Input: part model. Units: mm. Frame: model coordinates. Face numbers are marked on the shaded views. A direction names the side the tool comes from. Coordinates: 2 decimals unless noted, no trailing zeros. Loops run counter-clockwise (first coordinate to the right, second up) from the corner with the lowest first, then second, coordinate; pieces in that order, holes last. Notation, with made-up numbers: (37, 79.25) -> (58, 79.25) arc R11 ccw to (58, 83.25) -> close; hole circle Ø11 at (88.25, 81.5). An arc over 180 degrees is marked (long way). Answer as a JSON object with one key per item and string values.
from build123d import *

# Parameters (mm, degrees)
CROQUIS1_W                = 30
CROQUIS1_H                = 30
SALIENTE_EXTRUIR1_DEPTH   = 3
CROQUIS2_W                = 15
CROQUIS2_H                = 30
SALIENTE_EXTRUIR3_DEPTH   = 3
SALIENTE_EXTRUIR3_2_DEPTH = 3
CROQUIS3_W                = 30
CROQUIS3_H                = 30
SALIENTE_EXTRUIR4_DEPTH   = 3
SALIENTE_EXTRUIR5_DEPTH   = 3
CORTAR_EXTRUIR1_DEPTH     = 6
SALIENTE_EXTRUIR8_DEPTH   = 11
CROQUIS7_W                = 30
CROQUIS7_H                = 3.175
CORTAR_EXTRUIR3_DEPTH     = 18.542
CROQUIS9_W                = 60
CROQUIS9_H                = 0.175
SALIENTE_EXTRUIR9_DEPTH   = 11
CROQUIS10_W               = 90
CROQUIS10_H               = 5
CORTAR_EXTRUIR5_DEPTH     = 93
CROQUIS11_W               = 30
CROQUIS11_H               = 3.175
SALIENTE_EXTRUIR10_DEPTH  = 11
CROQUIS12_W               = 60
CROQUIS12_H               = 0.175
CORTAR_EXTRUIR6_DEPTH     = 11
CROQUIS13_W               = 30
CROQUIS13_H               = 5
CORTAR_EXTRUIR7_DEPTH     = 10
SALIENTE_EXTRUIR11_DEPTH  = 5


with BuildPart() as part:
    # Croquis1 → Saliente-Extruir1 (new body)
    with BuildSketch(Plane(origin=(0, 0, 0), x_dir=(1, 0, 0), z_dir=(0, 1, 0))):
        Rectangle(CROQUIS1_W, CROQUIS1_H)
    extrude(amount=SALIENTE_EXTRUIR1_DEPTH)



with BuildPart() as body_2:
    # Croquis2 → Saliente-Extruir3 (new body)
    with BuildSketch(Plane(origin=(0, 3, 0), x_dir=(1, 0, 0), z_dir=(0, 1, 0))):
        with Locations((-22.5, -30)):
            Rectangle(CROQUIS2_W, CROQUIS2_H)
    extrude(amount=-SALIENTE_EXTRUIR3_DEPTH)


with BuildPart() as body_3:
    # Croquis2 → Saliente-Extruir3 2 (new body)
    with BuildSketch(Plane(origin=(0, 3, 0), x_dir=(1, 0, 0), z_dir=(0, 1, 0))):
        with Locations((22.5, -30)):
            Rectangle(CROQUIS2_W, CROQUIS2_H)
    extrude(amount=-SALIENTE_EXTRUIR3_2_DEPTH)


with BuildPart() as part_1:
    add(part.part)

    add(body_2.part)  # Saliente-Extruir4 merges body 2

    add(body_3.part)  # Saliente-Extruir4 merges body 3
    # Croquis3 → Saliente-Extruir4 (add)
    with BuildSketch(Plane(origin=(0, 3, 0), x_dir=(1, 0, 0), z_dir=(0, 1, 0))):
        with Locations((0, -30)):
            Rectangle(CROQUIS3_W, CROQUIS3_H)
    extrude(amount=-SALIENTE_EXTRUIR4_DEPTH)

    # Croquis4 → Saliente-Extruir5 (add)
    with BuildSketch(Plane(origin=(0, 3, 0), x_dir=(1, 0, 0), z_dir=(0, 1, 0))):
        Polygon((-30, 0), (-45, 0), (-45, -60), (45, -60), (45, 0), (30, 0), (30, 30), (-30, 30), align=None)
    extrude(amount=SALIENTE_EXTRUIR5_DEPTH)

    # Croquis5 → Cortar-Extruir1 (cut)
    with BuildSketch(Plane(origin=(0, 0, 0), x_dir=(-1, 0, 0), z_dir=(0, -1, 0))):
        Polygon((30, -45), (30, -15), (15, -15), (15, 15), (-15, 15), (-15, -15), (-30, -15), (-30, -45), align=None)
    extrude(amount=-CORTAR_EXTRUIR1_DEPTH, mode=Mode.SUBTRACT)

    # Croquis6 → Saliente-Extruir8 (add)
    with BuildSketch(Plane(origin=(0, 3, 0), x_dir=(-1, 0, 0), z_dir=(0, -1, 0))):
        with BuildLine():
            Line((37.5, 0), (45, 0))
            Line((45, 0), (45, -60))
            Line((45, -60), (-45, -60))
            Line((-45, -60), (-45, 0))
            Line((-45, 0), (-37.5, 0))
            ThreePointArc((-37.5, 0), (-32.196699141, 2.196699141), (-30, 7.5))
            Line((-30, 7.5), (-30, 30))
            Line((-30, 30), (30, 30))
            Line((30, 30), (30, 7.5))
            ThreePointArc((30, 7.5), (32.196699141, 2.196699141), (37.5, 0))
        make_face()
        Polygon((15, 15), (15, -15), (30, -15), (30, -45), (-30, -45), (-30, -15), (-15, -15), (-15, 15), align=None, mode=Mode.SUBTRACT)
    extrude(amount=-SALIENTE_EXTRUIR8_DEPTH)

    # Croquis7 → Cortar-Extruir3 (cut)
    with BuildSketch(Plane(origin=(0, 14, 0), x_dir=(1, 0, 0), z_dir=(0, 1, 0))):
        with Locations((0, 16.5875)):
            Rectangle(CROQUIS7_W, CROQUIS7_H)
    extrude(amount=-CORTAR_EXTRUIR3_DEPTH, mode=Mode.SUBTRACT)

    # Croquis9 → Saliente-Extruir9 (add)
    with BuildSketch(Plane(origin=(0, 14, 0), x_dir=(1, 0, 0), z_dir=(0, 1, 0))):
        with Locations((0, 30.0875)):
            Rectangle(CROQUIS9_W, CROQUIS9_H)
    extrude(amount=-SALIENTE_EXTRUIR9_DEPTH)

    # Croquis10 → Cortar-Extruir5 (cut)
    with BuildSketch(Plane.XY.offset(60)):
        with Locations((0, 5.5)):
            Rectangle(CROQUIS10_W, CROQUIS10_H)
    extrude(amount=-CORTAR_EXTRUIR5_DEPTH, mode=Mode.SUBTRACT)

    # Croquis11 → Saliente-Extruir10 (add)
    with BuildSketch(Plane(origin=(0, 14, 0), x_dir=(1, 0, 0), z_dir=(0, 1, 0))):
        with Locations((0, 16.5875)):
            Rectangle(CROQUIS11_W, CROQUIS11_H)
    extrude(amount=-SALIENTE_EXTRUIR10_DEPTH)

    # Croquis12 → Cortar-Extruir6 (cut)
    with BuildSketch(Plane(origin=(0, 14, 0), x_dir=(1, 0, 0), z_dir=(0, 1, 0))):
        with Locations((0, 30.0875)):
            Rectangle(CROQUIS12_W, CROQUIS12_H)
    extrude(amount=-CORTAR_EXTRUIR6_DEPTH, mode=Mode.SUBTRACT)

    # Croquis13 → Cortar-Extruir7 (cut)
    with BuildSketch(Plane.XY.offset(-15)):
        with Locations((0, 5.5)):
            Rectangle(CROQUIS13_W, CROQUIS13_H)
    extrude(amount=-CORTAR_EXTRUIR7_DEPTH, mode=Mode.SUBTRACT)

    # Croquis14 → Saliente-Extruir11 (add)
    with BuildSketch(Plane(origin=(0, 14, 0), x_dir=(1, 0, 0), z_dir=(0, 1, 0))):
        with BuildLine():
            Line((-37.5, 0), (-45, 0))
            Line((-45, 0), (-45, -60))
            Line((-45, -60), (45, -60))
            Line((45, -60), (45, 0))
            Line((45, 0), (37.5, 0))
            ThreePointArc((37.5, 0), (32.196699141, 2.196699141), (30, 7.5))
            Line((30, 7.5), (30, 30))
            Line((30, 30), (-30, 30))
            Line((-30, 30), (-30, 7.5))
            ThreePointArc((-30, 7.5), (-32.196699141, 2.196699141), (-37.5, 0))
        make_face()
        Polygon((-15, 15), (-15, -15), (-30, -15), (-30, -45), (30, -45), (30, -15), (15, -15), (15, 15), align=None, mode=Mode.SUBTRACT)
    extrude(amount=SALIENTE_EXTRUIR11_DEPTH)


solid = part_1.part
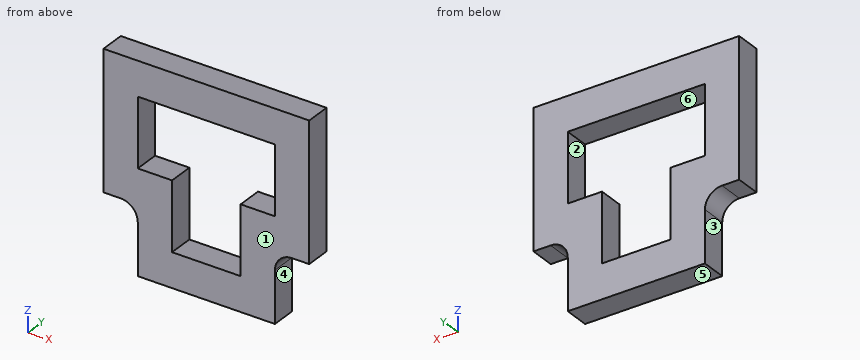
1. Section query A-A (x = -20.5). Return loops of the section in (y, z), plus the area to 3 significant figures.
Reply:
{"outline": "(8, -30) -> (19, -30) -> (19, 15) -> (8, 15) -> close; (8, 45) -> (19, 45) -> (19, 60) -> (8, 60) -> close", "area": "660 mm2"}
2. Section query C-C (y = 12.25). Return loops of the section in (x, z).
Reply:
{"outline": "(-45, 0) -> (-37.5, 0) arc R7.5 cw to (-30, -7.5) -> (-30, -30) -> (30, -30) -> (30, -7.5) arc R7.5 cw to (37.5, 0) -> (45, 0) -> (45, 60) -> (-45, 60) -> close; hole (-30, 15) -> (-15, 15) -> (-15, -15) -> (15, -15) -> (15, 15) -> (30, 15) -> (30, 45) -> (-30, 45) -> close"}
3. Section query B-B (z = 12). Return loops of the section in (x, y), plus the area to 3 significant figures.
Reply:
{"outline": "(-45, 8) -> (-15, 8) -> (-15, 19) -> (-45, 19) -> close; (15, 8) -> (45, 8) -> (45, 19) -> (15, 19) -> close", "area": "660 mm2"}
4. Pin query (flat end, axial travel): P1, Ø4, axis at y = 12.5, z = -13, coming from the +X side; P2, Ø4, axis at x = -34, y = 10, coming from the -Z side; P3, Ø6, axis at x = 40.5, y = 13, coming from the -Z side. Return the tip coordinate at first contact, or that it passes through.
Reply:
{"P1": "stops at x = 30", "P2": "stops at z = -2.4", "P3": "stops at z = 0"}
5. Mould query, pull axis X, two halves, no side actions, for the marked faces 1, 2 and 3. Classes: pulls with the +X half, pulls with the -X half, needs draft (parallel to the pull), parting line crosses it, or undercut.
Reply:
{"face 1": "needs draft", "face 2": "undercut", "face 3": "pulls with the -X half"}
6. Section query D-D (x = -39). Return loops of the section in (y, z).
Reply:
{"outline": "(8, 0) -> (19, 0) -> (19, 60) -> (8, 60) -> close"}
7. Line query: line 1 along X through (y, z) = (15.75, 4); line 2 along Z through (x, y) = (-21, 12.5); line 3 along Z through (x, y) = (9.5, 16). Output: solid intervals per line, ascending.
Reply:
{"line 1": "x = -45 to -15, 15 to 45", "line 2": "z = -30 to 15, 45 to 60", "line 3": "z = -30 to -15, 45 to 60"}
8. Access query for the marked faces 4, 5 and 6. Directions: +Z, -Z, +X, -X, +Y, -Y. A direction counts if a zero-diameter tool reaches every point of the face in a straight line with its end or side. Return the directions, or none.
Reply:
{"face 4": "-Z, +X, +Y, -Y", "face 5": "-Z, +X, -X, +Y, -Y", "face 6": "+Y, -Y"}
